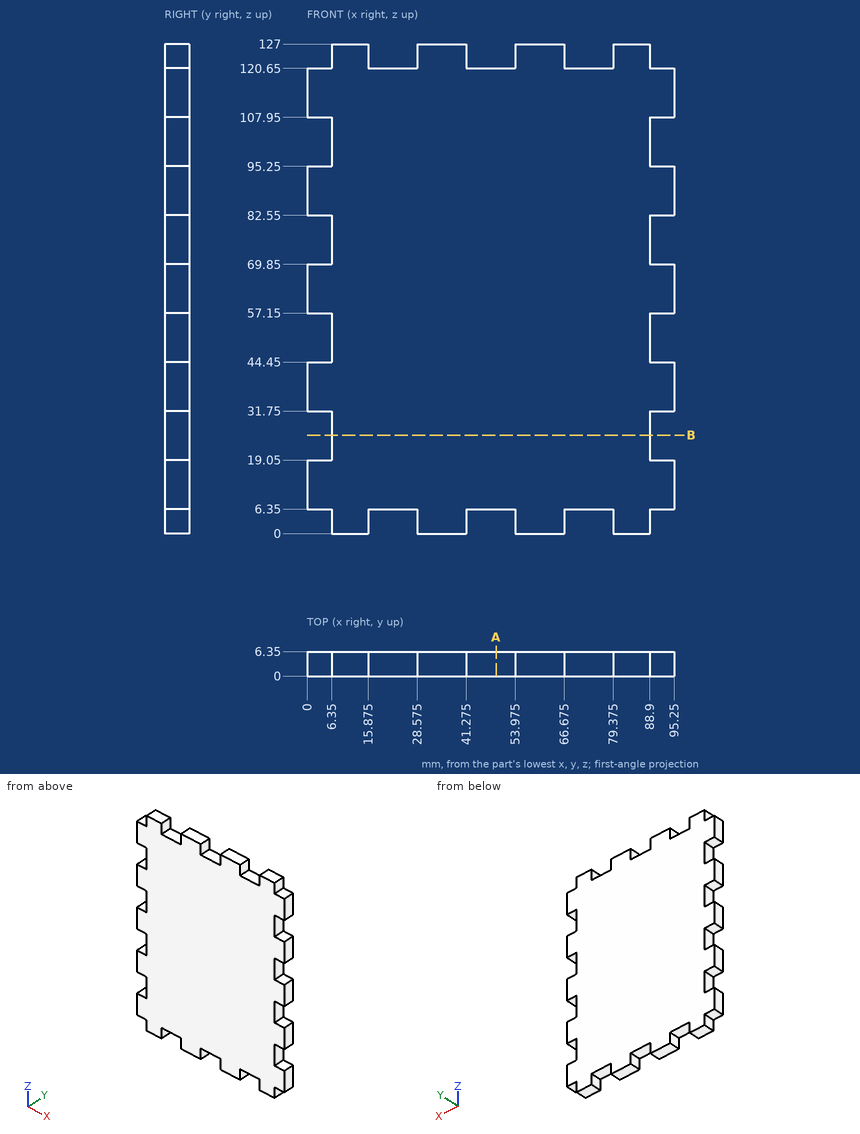
Study the drawing (mm; zero at the part's minimum x, y, z) and answer. Give positions to 0.01 mm unless a question says otherwise; leave off trailing zeros. Write each loop counter-clockwise with the first axis right and the second up, starting at its lowest first coordinate (ties: lowest second). Pieces come first, ordered by that corner, then holes. Notation, with made-up numbers: (-2, 78.5) - (25, 78.5) arc R15 ccw to (25, 86.5) - close; hole circle Ø6 at (28, -25). An arc over 180 degrees is marked (long way). One line per question, with ' | ' between items. Start each with the question number.
1. Section A-A, the plane x = 49 is taken. Determine the outline of the cut face in (y, z), then the cut area to 3 significant figures.
2. Section B-B, the plane z = 25.5 is taken. Determine the outline of the cut face in (x, y).
3. Given P1, Ø3, axis at x = 72.5, y = 2, coming from the -Z side; P2, Ø1.9, axis at x = 93, y = 4.5, coming from the +Z side; P3, Ø3, axis at y = 2, z = 48, coming from the -X side; P4, Ø2, axis at x = 30.5, y = 4, coming from the -Z side, each flat-ended and moving along its own axis, determine where each tip first touches the part or whether it passes through.
4. Straight lines are drawn through the part: line 1 (X direction, y = 5, z = 98); line 2 (Z direction, x = 23, y = 4.75). For each, find the intervals that lie inside material, in ascending order.
Result:
1) outline: (0, 6.35) - (6.35, 6.35) - (6.35, 120.65) - (0, 120.65) - close | area: 726 mm2
2) outline: (6.35, 0) - (88.9, 0) - (88.9, 6.35) - (6.35, 6.35) - close
3) P1: stops at z = 6.35 | P2: stops at z = 120.65 | P3: stops at x = 6.35 | P4: stops at z = 0
4) line 1: x = 6.35 to 88.9 | line 2: z = 6.35 to 120.65
